CAD build for the part. Positions are in the model's coordinates, mm. A direction names the side the tool comes from. Round coordinates to 2 decimals unless told otherwise and drop trailing zeros. Write each loop counter-clockwise with the first axis right and the second up, starting at its lowest first coordinate (ties: lowest second). Pieces come first, ordered by that corner, then holes. Notation, with made-up numbers: (88, 70) -> (137, 70) arc R35 ccw to (137, 104) -> close; hole circle Ø8 at (-19, 82). An arc over 180 degrees is marked (long way). Answer in a Markdown table with one row per item. Add a question column.
```python
from build123d import *

# Parameters (mm, degrees)
F1_DEPTH = 914.4
F3_DEPTH = 76.2


# Not quite as in the source:
# - a pattern or mirror of a feature is missing from the dataset's text; its kind, count and spacing are read off the source's solid


with BuildPart() as f1:
    # F0 (on Right) → F1 (new body, symmetric)
    with BuildSketch(Plane.YZ):
        with BuildLine():
            Line((-50.8, 0), (0, 0))
            ThreePointArc((0, 0), (-0.9299359697, 2.2450640303), (-3.175, 3.175))
            Line((-3.175, 3.175), (-47.625, 3.175))
            Line((-47.625, 3.175), (-47.625, 47.625))
            ThreePointArc((-47.625, 47.625), (-48.5549359697, 49.8700640303), (-50.8, 50.8))
            Line((-50.8, 50.8), (-50.8, 0))
        make_face()
    extrude(amount=F1_DEPTH, both=True)

    # F2 (on face) → F3 (cut)
    with BuildSketch(Plane(origin=(0, 0, 0), x_dir=(1, 0, 0), z_dir=(0, 0, -1))):
        Polygon((914.4, 50.8), (863.6, 0), (914.4, 0), align=None)
    f3 = extrude(amount=-F3_DEPTH, mode=Mode.SUBTRACT)

    # F3_copies: F3 across plane
    add(f3.mirror(Plane(origin=(0, 0, 0), x_dir=(0, 0, -1), z_dir=(-1, 0, 0))), mode=Mode.SUBTRACT)


solid = f1.part
```
Item 1: Saw through at B-B on y = -34.5. Give the cut face in (x, z) (3 decimals), then the cut area to 3 significant figures.
Item 2: Saw through at A-A on x = -107. Give the cut face in (y, z) (3 decimals).
Item 3: Pin check, flat tips, straight feed: pin 1 (5 mm diameter, centred on x = 213, y = -9, fed in from +Z) (3 decimals); pin 2 (5 mm diameter, centred on x = 305, z = 37.5, fed in from +Y) (3 decimals). Stop position of each tip, or through.
Item 4: Saw through at C-C on z = 29.5. Give the cut face in (x, y) (3 decimals), then the cut area to 3 significant figures.
Item 5: Drill centre lines: probe 1 along Y at (x, z) = (-117, 49); probe 2 along Z at (x, y) = (690, -22) (3 decimals); probe 3 along Y at (x, z) = (533, 17.5) (3 decimals). Where is each one in solid material? Low to high.
Item 6: Tool access for faces 1 (the flat face through (13, -26, 0)), 2 (the flat face through (13, -47.625, 25)): list every direction of +Z, -Z, +X, -X, +Y, -Y with a clear straight run to the whole face (end or side of a thin tool).
Recorded:
| question | item | result |
|---|---|---|
| 1 | outline | (-898.1, 0) -> (898.1, 0) -> (898.1, 3.175) -> (-898.1, 3.175) -> close |
| 1 | area | 5,700 mm2 |
| 2 | outline | (-50.8, 0) -> (0, 0) arc R3.175 ccw to (-3.175, 3.175) -> (-47.625, 3.175) -> (-47.625, 47.625) arc R3.175 ccw to (-50.8, 50.8) -> close |
| 3 | pin 1 | z = 3.175 |
| 3 | pin 2 | y = -47.625 |
| 4 | outline | (-914.4, -50.8) -> (914.4, -50.8) -> (911.225, -47.625) -> (-911.225, -47.625) -> close |
| 4 | area | 5,800 mm2 |
| 5 | probe 1 | -50.8 to -47.94 |
| 5 | probe 2 | 0 to 3.175 |
| 5 | probe 3 | -50.8 to -47.625 |
| 6 | face 1 | -Z, +X, -X, +Y, -Y |
| 6 | face 2 | +Z, +X, -X, +Y |
